Source: three-view drawing plus pictorial views. Frame: mm from the lowest corner of the part. Give positions to 0.01 mm unless a question says otherwise; leave off trailing zeros. Order: outer loops, then holes, each group sorted by start corner. A loop starts at its lowest first (then second) coordinate and runs counter-clockwise, first axis right, second up. Notation, with made-up numbers: (-15.75, -36) -> (0.25, -36) arc R35 ccw to (0.25, -4) -> close; hole circle Ø9 at (-19.75, 41). An arc over 180 degrees is marked (long way). Answer in a Markdown table with one row per item.
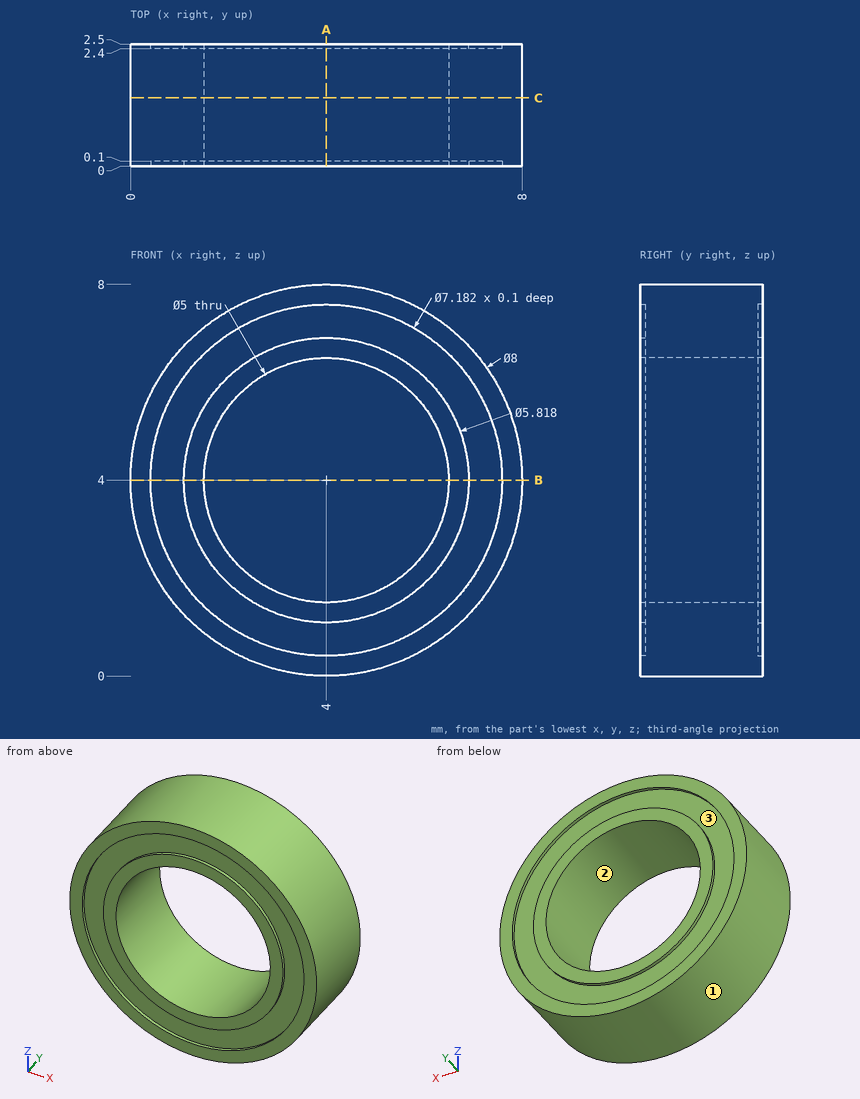
(1) Section query B-B (z = 4). Return the cut outline in (x, y).
A:
| item | result |
|---|---|
| outline | (0, 0) -> (0.41, 0) -> (0.41, 0.1) -> (1.09, 0.1) -> (1.09, 0) -> (1.5, 0) -> (1.5, 2.5) -> (1.09, 2.5) -> (1.09, 2.4) -> (0.41, 2.4) -> (0.41, 2.5) -> (0, 2.5) -> close; (6.5, 0) -> (6.91, 0) -> (6.91, 0.1) -> (7.59, 0.1) -> (7.59, 0) -> (8, 0) -> (8, 2.5) -> (7.59, 2.5) -> (7.59, 2.4) -> (6.91, 2.4) -> (6.91, 2.5) -> (6.5, 2.5) -> close |
(2) Section query A-A (x = 4). Return the cut outline in (y, z).
A:
| item | result |
|---|---|
| outline | (0, 0) -> (2.5, 0) -> (2.5, 0.41) -> (2.4, 0.41) -> (2.4, 1.09) -> (2.5, 1.09) -> (2.5, 1.5) -> (0, 1.5) -> (0, 1.09) -> (0.1, 1.09) -> (0.1, 0.41) -> (0, 0.41) -> close; (0, 6.5) -> (2.5, 6.5) -> (2.5, 6.91) -> (2.4, 6.91) -> (2.4, 7.59) -> (2.5, 7.59) -> (2.5, 8) -> (0, 8) -> (0, 7.59) -> (0.1, 7.59) -> (0.1, 6.91) -> (0, 6.91) -> close |
(3) Pull-direction query (Z, two-part tool) for the marked faces 1, 2 and 3; classes: +Z half, -Z half, draft (parallel to the pull), parting line (faces both ways), or undercut.
A:
| item | result |
|---|---|
| face 1 | parting line |
| face 2 | undercut |
| face 3 | undercut |
(4) Ray query, probe 1 along X at (y, z) = (1.2, 4); probe 2 along Y at (x, z) = (6.5, 2); probe 3 along Z at (x, y) = (4.5, 2.15). Return the intervals inside material, ascending.
A:
| item | result |
|---|---|
| probe 1 | x = 0 to 1.5, 6.5 to 8 |
| probe 2 | y = 0.1 to 2.4 |
| probe 3 | z = 0.03 to 1.55, 6.45 to 7.97 |
(5) First-contact query: pin 1 Ø1 at (y, z) = (1, 6) entering from -X; pin 2 Ø2 at (x, z) = (3.5, 4.5) entering from -Y. Flat tips, straight axial feed; report the tip coordinate or a pass-through.
A:
| item | result |
|---|---|
| pin 1 | stops at x = 0.29 |
| pin 2 | passes through |
(6) Section query C-C (y = 1.4). Return the cut outline in (x, z).
A:
| item | result |
|---|---|
| outline | circle Ø8 at (4, 4); hole circle Ø5 at (4, 4) |
